Autodesk Fusion 360 part; units mm, degrees
sketch "Front" plane through (0, 0, 0) normal (0, 1, 0) x (1, 0, 0) in component "2004699A"
  line L0 (-34.4613, 0.7342) -> (100.7673, 0.7342) construction
  line L1 (-34.854, -115.3184) -> (120.0108, -115.3184) construction
  line L2 (39.1093, -14.9122) -> (120.6654, -14.9122) construction
  line L3 (3.575, 24.5274) -> (3.575, -141.9882) construction
  line L4 (78.251, 23.8729) -> (78.251, -119.9956) construction
  line L5 (-16.7886, -108.2138) -> (88.0691, -108.2138) construction
  line L6 (-18.2286, -5.0898) -> (85.3201, -5.0898) construction
  line L7 (-8.6723, -56.6518) -> (96.0546, -56.6518) construction
  line L8 (-24.3813, -113.9722) -> (90.4255, -113.9722) construction
  line L9 (-27.0881, -0.4088) -> (83.5136, -0.4088) construction
  line L10 (10.2552, -130.527) -> (10.2552, 10.1996) construction
  line L11 (71.52, -130.1852) -> (71.52, 12.6775) construction
  line L12 (5.7848, -130.0998) -> (5.7848, 6.3546) construction
  line L13 (83.0008, -137.1267) -> (83.0008, 10.6162) construction
  line L14 (-1.2002, -137.339) -> (-1.2002, 17.644) construction
  line L15 (110.5413, -110.6956) -> (5.7848, -110.6956) construction
  line L16 (110.1974, -4.2696) -> (-2.9547, -4.2696) construction
  line L17 (102.8889, -60.7158) -> (-8.8875, -60.7158) construction
  line L18 (102.459, -52.5878) -> (-11.4669, -52.5878) construction
  line L19 (40.913, -17.1802) -> (40.913, 17.1835) construction
  line L20 (69.6478, 8.6501) -> (89.4046, -11.1067) construction
  line L21 (-5.4342, -8.9542) -> (10.2552, 6.7154) construction
  line L22 (-6.1303, -103.6453) -> (12.6902, -122.4658) construction
  line L23 (73.7302, -117.8806) -> (90.3753, -101.2137) construction
  line L24 (-2.868, -104.1498) -> (87.443, -104.1498) construction
  line L25 (-3.4391, -112.2778) -> (87.0011, -112.2778) construction
  line L26 (-3.1536, -9.1538) -> (86.0732, -9.1538) construction
  line L27 (-3.3677, -1.0258) -> (85.288, -1.0258) construction
  line L28 (10.2552, -110.6956) -> (71.52, -110.6956)
  line L29 (71.52, -110.6956) -> (71.52, -4.2696)
  line L30 (71.52, -4.2696) -> (10.2552, -4.2696)
  line L31 (10.2552, -4.2696) -> (10.2552, -110.6956)
  line L32 (-1.2002, -115.3184) -> (83.0008, -115.3184)
  line L33 (83.0008, -115.3184) -> (83.0008, 0.7342)
  line L34 (83.0008, 0.7342) -> (-1.2002, 0.7342)
  line L35 (-1.2002, 0.7342) -> (-1.2002, -115.3184)
  line L36 (76.0158, -119.9569) -> (76.0158, 9.6762) construction
  line L37 (5.7848, -115.3184) -> (76.0222, -115.3184) construction
  line L38 (76.0222, -115.3184) -> (76.0222, 0.7342) construction
  line L39 (76.0222, 0.7342) -> (5.7848, 0.7342) construction
  line L40 (5.7848, 0.7342) -> (5.7848, -115.3184) construction
  line L41 (76.0222, 0.7342) -> (5.7848, 0.7342)
  line L42 (5.7848, 0.7342) -> (5.7848, -115.3184)
  line L43 (5.7848, -115.3184) -> (76.0222, -115.3184)
  line L44 (76.0222, -115.3184) -> (76.0222, 0.7342)
  line L45 (-1.2002, -108.5588) -> (5.5429, -115.3184)
  line L46 (76.2891, -115.3184) -> (83.0008, -108.585)
  line L47 (77.5637, 0.7342) -> (83.0008, -4.7029)
  line L48 (4.2664, 0.7342) -> (-1.2002, -4.7255)
  point P0 (3.575, -108.2138)
  point P1 (78.251, -108.2138)
  point P2 (78.251, -56.6518)
  point P3 (78.251, -5.0898)
  point P4 (3.575, -5.0898)
  point P5 (3.575, -56.6518)
  dimension "d1" = 1.143
  dimension "d2" = 116.0526
  dimension "d3" = 113.5634
  dimension "d4" = 103.124
  dimension "d5" = 51.562
  dimension "d6" = 74.676
  dimension "d7" = 2.2098
  dimension "d8" = 4.4704
  dimension "d9" = 61.2648
  dimension "d10" = 84.201
  dimension "d11" = 6.985
  dimension "d12" = 106.426
  dimension "d13" = 4.6228
  dimension "d14" = 100.4062
  dimension "d15" = 37.338
  dimension "d16" = 8.128
  dimension "d17" = 4.064
  dimension "d18" = 3.6322
  dimension "d19" = 3.6322
  dimension "d20" = 3.6322
  dimension "d21" = 3.6322
  dimension "d22" = 4.064
  dimension "d23" = 8.128
  dimension "d25" = 4.064
  dimension "d26" = 8.128
  dimension "d27" = 70.231
extrude "Extrude1" add sketch "Front" against normal blind 17.0434 contours L32 L34 L41 L42 L43 L44 in component "2004699A"
extrude "Extrude2" add sketch "Front" against normal blind 2.0828 contours L32 L34 L35 L42 L45 L48 | L32 L33 L34 L44 L46 L47 in component "2004699A"
fillet "Fillet1" radius 4.318 4 edges at (5.7848, -9.5631, -0.7342) (76.0222, -9.5631, -0.7342) (76.0222, -9.5631, 115.3184) (5.7848, -9.5631, 115.3184) in component "2004699A"
fillet "Fillet2" radius 2.8194 4 edges at (71.52, -8.5217, 110.6956) (10.2552, -8.5217, 110.6956) (71.52, -8.5217, 4.2696) (10.2552, -8.5217, 4.2696) in component "2004699A"
hole "Hole1" at (78.251, 0, 108.2138) at (78.251, 0, 56.6518) at (78.251, 0, 5.0898) at (3.575, 0, 5.0898) at (3.575, 0, 56.6518) at (3.575, 0, 108.2138) direction (0, -1, 0) diameter 4.3434 end through all in component "2004699A"
sketch "Sketch3" plane through (0, 0, 0) normal (0, 1, 0) x (1, 0, 0) in component "2004699A"
  line L0 (88.5571, -114.1754) -> (-29.017, -114.1754) construction
  line L1 (6.9278, -119.135) -> (6.9278, -3.6092) construction
  line L2 (74.8728, -110.975) -> (74.8728, 6.1599) construction
  line L3 (95.5329, -0.4088) -> (-26.782, -0.4088) construction
  line L4 (-34.4613, 0.7342) -> (100.7673, 0.7342) construction
  line L5 (5.7848, -130.0998) -> (5.7848, 6.3546) construction
  line L6 (-34.854, -115.3184) -> (120.0108, -115.3184) construction
  line L7 (76.0158, -119.9569) -> (76.0158, 9.6762) construction
  line L8 (71.6724, -114.1754) -> (10.1282, -114.1754)
  line L9 (6.9278, -110.975) -> (6.9278, -0.4088)
  line L10 (10.1282, -0.4088) -> (71.6724, -0.4088)
  line L11 (74.8728, -3.6092) -> (74.8728, -114.1754)
  arc A0 (74.8728, -3.6092) -> (71.6724, -0.4088) centre (71.6724, -3.6092) ccw
  arc A1 (10.1282, -0.4088) -> (6.9278, -3.6092) centre (10.1282, -3.6092) ccw
  arc A2 (71.6724, -114.1754) -> (74.8728, -110.975) centre (71.6724, -110.975) ccw
  arc A3 (6.9278, -110.975) -> (10.1282, -114.1754) centre (10.1282, -110.975) ccw
  dimension "d37" = 1.143
  dimension "d38" = 1.143
  dimension "d39" = 1.143
  dimension "d40" = 1.143
  dimension "d41" = 3.2004
  dimension "d42" = 3.2004
  dimension "d43" = 3.2004
  dimension "d44" = 3.2004
extrude "Extrude3" cut sketch "Sketch3" against normal blind 14.986 in component "2004699A"
chamfer "Chamfer1" distance 2.032 angle 45 8 edges at (40.8876, -14.986, 4.2696) (11.081, -14.986, 5.0954) (10.2552, -14.986, 57.4826) (11.081, -14.986, 109.8698) (40.8876, -14.986, 110.6956) (70.6942, -14.986, 109.8698) (71.52, -14.986, 57.4826) (70.6942, -14.986, 5.0954) in component "2004699A"
sketch "Sketch4" plane through (83.0008, 0, 0) normal (1, 0, 0) x (0, 1, 0) in component "2004699A"
  line L0 (0, 4.7029) -> (0, 108.585)
  line L1 (0, 108.585) -> (-2.0828, 108.585)
  line L2 (-2.0828, 108.585) -> (-2.0828, 4.7029)
  line L3 (-2.0828, 4.7029) -> (0, 4.7029)
  line L4 (-0.9906, 121.8672) -> (-0.9906, -5.2486) construction
  line L5 (0, 108.2121) -> (-3.3976, 108.2121) construction
  line L6 (0, 56.644) -> (-3.817, 56.644) construction
  line L7 (0, 0) -> (-1.1062, 0) construction
  line L8 (1.8872, 112.2761) -> (-9.9271, 112.2761) construction
  line L9 (1.8112, 104.1481) -> (-10.4595, 104.1481) construction
  line L10 (1.71, 60.708) -> (-9.8241, 60.708) construction
  line L11 (2.1656, 52.58) -> (0.9254, 52.58) construction
  line L12 (0.9254, 52.58) -> (-9.5412, 52.58) construction
  line L13 (0, 5.0822) -> (-6.1548, 5.0822) construction
  line L14 (2.1892, 9.1462) -> (-10.0058, 9.1462) construction
  line L15 (2.6197, 1.0182) -> (-10.581, 1.0182) construction
  line L16 (-8.6106, 122.6091) -> (-8.6106, -10.4565) construction
  line L17 (-8.6106, 60.708) -> (-0.9906, 60.708)
  line L18 (-0.9906, 60.708) -> (-0.9906, 52.58)
  line L19 (-0.9906, 52.58) -> (-8.6106, 52.58)
  line L20 (-8.6106, 52.58) -> (-8.6106, 60.708)
  line L21 (-8.6106, 9.1462) -> (-0.9906, 9.1462)
  line L22 (-0.9906, 9.1462) -> (-0.9906, 1.0182)
  line L23 (-0.9906, 1.0182) -> (-8.6106, 1.0182)
  line L24 (-8.6106, 1.0182) -> (-8.6106, 9.1462)
  line L25 (-8.6106, 112.2761) -> (-0.9906, 112.2761)
  line L26 (-0.9906, 112.2761) -> (-0.9906, 104.1481)
  line L27 (-0.9906, 104.1481) -> (-8.6106, 104.1481)
  line L28 (-8.6106, 104.1481) -> (-8.6106, 112.2761)
  point P0 (0, 119.9956)
  dimension "d48" = 0.9906
  dimension "d49" = 4.064
  dimension "d50" = 8.128
  dimension "d51" = 4.064
  dimension "d52" = 8.128
  dimension "d54" = 4.064
  dimension "d55" = 8.128
  dimension "d56" = 7.62
extrude "Extrude4" cut sketch "Sketch4" against normal through all contours L2 L3 L21 L22 L23 L24 | L2 L3 L21 L22 | L1 L2 L26 L27 | L1 L2 L25 L26 L27 L28 | L2 L17 L19 L20 | L2 L17 L18 L19 in component "2004699A"
component "2004699A" placed x (1, 0, 0) y (0, 1, 0) z (0, 0, 1) at (0, 0, 0)
equation "d41 = 0.171 in - 0.045 in"
equation "d42 = 0.171 in - 0.045 in"
equation "d43 = 0.171 in - 0.045 in"
equation "d44 = 0.171 in - 0.045 in"
Input: part model. Units: mm. Frame: model coordinates. A direction names the side the tool comes from. Round coordinates to 2 decimals unless told otherwise and drop trailing zeros. Write each loop counter-clockwise with the first axis right and the second up, starting at its lowest first coordinate (ties: lowest second). Pieces come first, ordered by that corner, then holes. Notation, with made-up numbers: M 58,-31.75 L 115,-31.75 A33 cw 115,-1.75 Z; hole C 43,-27.75 d6. An arc over 180 degrees is marked long. Write each question's results on one line, items separated by ' | '.
Q1. Pin query (flat end, axial travel): P1, Ø3.5, axis at x = 1, z = 91.5, coming from the -Y side; P2, Ø2, axis at y = -13, z = 96, coming from the -X side; P3, Ø8, axis at y = -15, z = 55, coming from the +X side. Return the tip coordinate at first contact, or that it passes through.
Results:
P1: stops at y = -2.08 | P2: stops at x = 5.78 | P3: stops at x = 76.02
Q2. Section query D-D (z = 56.5). State how many separate pieces and enclosed holes the cut face has, and give its area (3 significant figures).
Results:
separate pieces: 6 | enclosed holes: 0 | area: 36.5 mm^2
Q3. Draft query along Z for faces 4 (the face through (41, -8, -0.734)), 5 (the face through (6.3, -3.7, 112.276)), 6 (the face through (5.785, -9, 57)). Return one class per face: released by +Z, released by -Z, zero draft, split by the parting line, or undercut.
Results:
face 4: released by -Z | face 5: undercut | face 6: zero draft
Q4. Access query for faces 1 (the face through (77.5, -1.7, 52.58)), 2 (the face through (79, -2.083, 31)), 3 (the face through (73.91, -7.388, 113.263)). Directions: +Z, -Z, +X, -X, +Y, -Y. A direction counts if a zero-diameter tool reaches every point of the face in a straight line with its end or side. Return the directions, or none.
Results:
face 1: +X, -X | face 2: +Z, -Z, +X, -Y | face 3: +Y
Q5. Section query B-B (y = -12.75). Return loops of the section in (x, z) (3 decimals).
Results:
outline: M 5.785,3.584 A4.318 ccw 10.103,-0.734 L 71.704,-0.734 A4.318 ccw 76.022,3.584 L 76.022,111 A4.318 ccw 71.704,115.318 L 10.103,115.318 A4.318 ccw 5.785,111 Z; hole M 6.928,3.609 A3.2 ccw 10.128,0.409 L 71.672,0.409 A3.2 ccw 74.873,3.609 L 74.873,110.975 A3.2 ccw 71.672,114.175 L 10.128,114.175 A3.2 ccw 6.928,110.975 Z
Q6. Line query: line 1 along Z through (x, y) = (50, -14.5); line 2 along X through (y, z) = (-12, 25.5); line 3 along X through (y, z) = (-1, 21). Output: solid intervals per line, ascending.
Results:
line 1: z = -0.73 to 0.41, 114.18 to 115.32 | line 2: x = 5.78 to 6.93, 74.87 to 76.02 | line 3: x = -1.2 to 6.93, 74.87 to 83
